Part model, mm, in its own coordinate system. A direction names the side the tool comes from. Round coordinates to 2 decimals unless told otherwise and drop trailing zeros. Order: outer loops, then holes, each group sorted by start corner. A loop starts at its lowest first (then second) coordinate and runs counter-clockwise, first axis right, second up. Notation, with made-up numbers: (-25.75, 57.25) -> (24.25, 57.25) arc R24 ccw to (24.25, 89.25) -> close; hole circle Ø6 at (52, -28.75). An arc over 180 degrees is marked (long way). Use CSV: the item, a comma, the result in double quotes.
```python
from build123d import *
from build123d.topology import SkipClean

# Parameters (mm, degrees)
BOSS_EXTRUDE1_DEPTH     = 93
SKETCH1_4_R             = 39
SKETCH1_4_R_2           = 29
EXTRUDE_THIN1_DEPTH     = 93
CUT_EXTRUDE_THIN1_DEPTH = 76


# Read off the part's stored shape, not the designer's step: Cut-Extrude-Thin1
with BuildPart() as part:
    # Sketch1 → Boss-Extrude1 (new body)
    with BuildSketch(Plane(origin=(0, 0, 0), x_dir=(1, 0, 0), z_dir=(0, 1, 0))):
        with BuildLine():
            Line((-86.602540378, -50), (-25.11473671, -14.5))
            ThreePointArc((-25.11473671, -14.5), (-26.712107385, -11.289965415), (-27.901144427, -7.907347195))
            Line((-27.901144427, -7.907347195), (-89.935126387, -43.722683378))
            ThreePointArc((-89.935126387, -43.722683378), (-88.324617875, -46.890957308), (-86.602540378, -50))
        make_face()
        with BuildLine():
            ThreePointArc((-20.798535761, -20.209426271), (-23.133450549, -17.488380876), (-25.11473671, -14.5))
            Line((-25.11473671, -14.5), (-86.602540378, -50))
            ThreePointArc((-86.602540378, -50), (-84.771069174, -53.045884205), (-82.83251772, -56.024762455))
            Line((-82.83251772, -56.024762455), (-20.798535761, -20.209426271))
        make_face()
        with BuildLine():
            ThreePointArc((27.901144427, -7.907347195), (26.712107385, -11.289965415), (25.11473671, -14.5))
            Line((25.11473671, -14.5), (86.602540378, -50))
            ThreePointArc((86.602540378, -50), (88.324617875, -46.890957308), (89.935126387, -43.722683378))
            Line((89.935126387, -43.722683378), (27.901144427, -7.907347195))
        make_face()
        with BuildLine():
            Line((86.602540378, -50), (25.11473671, -14.5))
            ThreePointArc((25.11473671, -14.5), (23.133450549, -17.488380876), (20.798535761, -20.209426271))
            Line((20.798535761, -20.209426271), (82.83251772, -56.024762455))
            ThreePointArc((82.83251772, -56.024762455), (84.771069174, -53.045884205), (86.602540378, -50))
        make_face()
        with BuildLine():
            ThreePointArc((-7.102608667, 28.116773466), (-3.578656835, 28.778346291), (0, 29))
            Line((0, 29), (0, 100))
            ThreePointArc((0, 100), (-3.553548701, 99.936841513), (-7.102608667, 99.747445833))
            Line((-7.102608667, 99.747445833), (-7.102608667, 28.116773466))
        make_face()
        with BuildLine():
            Line((0, 100), (0, 29))
            ThreePointArc((0, 29), (3.578656835, 28.778346291), (7.102608667, 28.116773466))
            Line((7.102608667, 28.116773466), (7.102608667, 99.747445833))
            ThreePointArc((7.102608667, 99.747445833), (3.553548701, 99.936841513), (0, 100))
        make_face()
    extrude(amount=BOSS_EXTRUDE1_DEPTH)

    # Sketch1<4> → Extrude-Thin1 (add)
    with SkipClean():  # the faces are left unmerged after this step: merging them gives an invalid solid
        with BuildSketch(Plane(origin=(0, 0, 0), x_dir=(1, 0, 0), z_dir=(0, 1, 0))):
            Circle(SKETCH1_4_R)
            Circle(SKETCH1_4_R_2, mode=Mode.SUBTRACT)
        extrude(amount=EXTRUDE_THIN1_DEPTH)

    # Cut-Extrude-Thin1 outline → Cut-Extrude-Thin1 (cut)
    with SkipClean():  # the faces are left unmerged after this step: merging them gives an invalid solid
        with BuildSketch(Plane(origin=(0, 0, 0), x_dir=(1, 0, 0), z_dir=(0, 1, 0))):
            with BuildLine():
                Line((2, 28.930952283), (2, 99.979998))
                ThreePointArc((2, 99.979998), (0, 100), (-2, 99.979998))
                Line((-2, 99.979998), (-2, 28.930952283))
                ThreePointArc((-2, 28.930952283), (0, 29), (2, 28.930952283))
            make_face()
            with BuildLine():
                Line((87.585218138, -48.257948192), (26.054939633, -12.733425334))
                ThreePointArc((26.054939633, -12.733425334), (25.11473671, -14.5), (24.054939633, -16.197526949))
                Line((24.054939633, -16.197526949), (85.585218138, -51.722049807))
                ThreePointArc((85.585218138, -51.722049807), (86.602540378, -50), (87.585218138, -48.257948192))
            make_face()
            with BuildLine():
                ThreePointArc((-24.054939633, -16.197526949), (-25.11473671, -14.5), (-26.054939633, -12.733425334))
                Line((-26.054939633, -12.733425334), (-87.585218138, -48.257948192))
                ThreePointArc((-87.585218138, -48.257948192), (-86.602540378, -50), (-85.585218138, -51.722049807))
                Line((-85.585218138, -51.722049807), (-24.054939633, -16.197526949))
            make_face()
        extrude(amount=CUT_EXTRUDE_THIN1_DEPTH, mode=Mode.SUBTRACT)


solid = part.part
```
(1) Cut at B-B, the plane x = 10. Give the cut face in (y, z).
Reply:
outline,"(0, -37.7) -> (93, -37.7) -> (93, -27.22) -> (0, -27.22) -> close; (0, 27.22) -> (93, 27.22) -> (93, 37.7) -> (0, 37.7) -> close"
(2) Cut at C-C, the plane z = -64. Give the cut face in (x, y).
Reply:
outline,"(-7.1, 0) -> (-2, 0) -> (-2, 76) -> (2, 76) -> (2, 0) -> (7.1, 0) -> (7.1, 93) -> (-7.1, 93) -> close"
(3) Probe probe 1 along X at (y, z) = (43, 35); probe 2 along X at (y, z) = (75, -86.5); probe 3 along X at (y, z) = (45.5, 22.5). List the from-to ranges inside material, lowest first. Write a range as [from, to].
Reply:
probe 1,"[-74.83, -64.62], [-56.62, -46.42], [-17.2, 17.2], [46.42, 56.62], [64.62, 74.83]"
probe 2,"[-7.1, -2], [2, 7.1]"
probe 3,"[-53.18, -42.97], [-34.97, -18.3], [18.3, 34.97], [42.97, 53.18]"
(4) Which spindle directions (+Z, -Z, +X, -X, +Y, -Y) get a long thin tool onto all of the face, cutting with end or side? Do faces 5 (the face through (-2, 37, -65)), 6 (the face through (-55.25, 37.47, 34.21)), 7 (the face through (-56.62, 45.85, 40.89)), 8 (the face through (7.103, 46, -69)). Say none if no direction does.
Reply:
face 5,"-Z, -Y"
face 6,"-Y"
face 7,"+Z, +Y, -Y"
face 8,"-Z, +X, +Y, -Y"
(5) Pull direction Z, two halves, no side cores. Call faces 1 (the face through (56, 76, 32)), 2 (the face through (-33.537, 45.849, -19.907)), 3 (the face through (0, 46, 39)), 4 (the face through (0, 76, -65)): released by +Z, released by -Z, zero draft, split by the parting line, or undercut.
Reply:
face 1,"undercut"
face 2,"undercut"
face 3,"released by +Z"
face 4,"zero draft"
(6) Cut at D-D, the plane x = 62. Give the cut face in (y, z).
Reply:
outline,"(0, 27.59) -> (93, 27.59) -> (93, 44) -> (0, 44) -> (0, 38.11) -> (76, 38.11) -> (76, 33.49) -> (0, 33.49) -> close"
(7) Cut at A-A, the plane y = 15. Give the cut face in (x, z), then the cut area to 3 significant figures.
Reply:
outline,"(-89.94, 43.72) -> (-36.76, 13.02) arc R39 ccw to (-7.1, -38.35) -> (-7.1, -99.75) arc R100 ccw to (-2, -99.98) -> (-2, -28.93) arc R29 cw to (-26.05, 12.73) -> (-87.59, 48.26) arc R100 ccw to start; (-85.59, 51.72) -> (-24.05, 16.2) arc R29 cw to (24.05, 16.2) -> (85.59, 51.72) arc R100 ccw to (82.83, 56.02) -> (29.66, 25.32) arc R39 ccw to (-29.66, 25.32) -> (-82.83, 56.02) arc R100 ccw to start; (2, -99.98) arc R100 ccw to (7.1, -99.75) -> (7.1, -38.35) arc R39 ccw to (36.76, 13.02) -> (89.94, 43.72) arc R100 ccw to (87.59, 48.26) -> (26.05, 12.73) arc R29 cw to (2, -28.93) -> close"
area,"3,890 mm2"
(8) Drop flat-ended pins along their axis: P1, Ø10, axis at y = 30, z = -26, coming from the -X side; P2, Ø2, axis at y = 81.5, z = -2.5, coming from the -X side; P3, Ø3, axis at y = 78, z = -57.5, coming from the +X side. Give the stop position or say it passes through.
Reply:
P1,"x = -32.86"
P2,"x = -38.97"
P3,"x = 7.1"
